from build123d import *

# Parameters (mm, degrees)
F1_DEPTH = 254
F2_DEPTH = 190.5
F3_DEPTH = 127
F4_DEPTH = 63.5
F5_R     = 12.6999
F6_R     = 25.3999
F7_R     = 12.6999


# Not quite as in the source:
# - a fillet or chamfer that OpenCascade refuses, or shapes differently, is made with other operations: its cross-section is extruded or revolved along the edge and cut away or added
# - a fillet or chamfer is up to 0.001 mm smaller than in the source, because OpenCascade refuses the exact size


with BuildPart() as f1:
    # F0 (on Right) → F1 (new body)
    with BuildSketch(Plane.YZ):
        with BuildLine():
            ThreePointArc((12.7, 0), (8.9802561211, 8.9802561211), (0, 12.7))
            ThreePointArc((0, 12.7), (-8.9802561211, 8.9802561211), (-12.7, 0))
            ThreePointArc((-12.7, 0), (-8.9802561211, -8.9802561211), (0, -12.7))
            ThreePointArc((0, -12.7), (8.9802561211, -8.9802561211), (12.7, 0))
        make_face()
    extrude(amount=F1_DEPTH)

    # F0 (on Right) → F2 (join)
    with BuildSketch(Plane.YZ):
        with BuildLine():
            ThreePointArc((-12.7, 0), (-8.9802561211, 8.9802561211), (0, 12.7))
            Line((0, 12.7), (-12.7, 12.7))
            Line((-12.7, 12.7), (-12.7, 0))
        make_face()
        with BuildLine():
            Line((12.7, 12.7), (0, 12.7))
            ThreePointArc((0, 12.7), (8.9802561211, 8.9802561211), (12.7, 0))
            Line((12.7, 0), (12.7, 12.7))
        make_face()
        with BuildLine():
            Line((12.7, -12.7), (12.7, 0))
            ThreePointArc((12.7, 0), (8.9802561211, -8.9802561211), (0, -12.7))
            Line((0, -12.7), (12.7, -12.7))
        make_face()
        with BuildLine():
            ThreePointArc((0, -12.7), (-8.9802561211, -8.9802561211), (-12.7, 0))
            Line((-12.7, 0), (-12.7, -12.7))
            Line((-12.7, -12.7), (0, -12.7))
        make_face()
    extrude(amount=F2_DEPTH)

    # F0 (on Right) → F3 (join)
    with BuildSketch(Plane.YZ):
        with BuildLine():
            ThreePointArc((25.4, 0), (17.9605122421, 17.9605122421), (0, 25.4))
            ThreePointArc((0, 25.4), (-17.9605122421, 17.9605122421), (-25.4, 0))
            ThreePointArc((-25.4, 0), (-17.9605122421, -17.9605122421), (0, -25.4))
            ThreePointArc((0, -25.4), (17.9605122421, -17.9605122421), (25.4, 0))
        make_face()
        Polygon((-12.7, 12.7), (0, 12.7), (12.7, 12.7), (12.7, 0), (12.7, -12.7), (0, -12.7), (-12.7, -12.7), (-12.7, 0), align=None, mode=Mode.SUBTRACT)
    extrude(amount=F3_DEPTH)

    # F0 (on Right) → F4 (join)
    with BuildSketch(Plane.YZ):
        with BuildLine():
            ThreePointArc((-25.4, 0), (-17.9605122421, 17.9605122421), (0, 25.4))
            Line((0, 25.4), (-25.4, 25.4))
            Line((-25.4, 25.4), (-25.4, 0))
        make_face()
        with BuildLine():
            ThreePointArc((0, -25.4), (-17.9605122421, -17.9605122421), (-25.4, 0))
            Line((-25.4, 0), (-25.4, -25.4))
            Line((-25.4, -25.4), (0, -25.4))
        make_face()
        with BuildLine():
            Line((25.4, -25.4), (25.4, 0))
            ThreePointArc((25.4, 0), (17.9605122421, -17.9605122421), (0, -25.4))
            Line((0, -25.4), (25.4, -25.4))
        make_face()
        with BuildLine():
            Line((25.4, 25.4), (0, 25.4))
            ThreePointArc((0, 25.4), (17.9605122421, 17.9605122421), (25.4, 0))
            Line((25.4, 0), (25.4, 25.4))
        make_face()
    extrude(amount=F4_DEPTH)

    # F5 (radius 12.7 in the source; OpenCascade refuses exactly that, so slightly less here)
    f5_edges = [f1.edges().sort_by_distance(p)[0] for p in [
        (158.75, -12.7, -12.7),
        (158.75, 12.7, -12.7),
        (158.75, 12.7, 12.7),
        (158.75, -12.7, 12.7),
    ]]
    fillet(f5_edges, radius=F5_R)

    # F6 (radius 25.4 in the source; OpenCascade refuses exactly that, so slightly less here)
    f6_edges = [f1.edges().sort_by_distance(p)[0] for p in [
        (31.75, -25.4, -25.4),
        (31.75, 25.4, -25.4),
        (31.75, -25.4, 25.4),
        (31.75, 25.4, 25.4),
    ]]
    fillet(f6_edges, radius=F6_R)

    # F7 (radius 12.7 in the source; OpenCascade refuses exactly that, so slightly less here)
    f7_edges = [f1.edges().sort_by_distance(p)[0] for p in [
        (127, 25.4, 0),
    ]]
    fillet(f7_edges, radius=F7_R)

    # F8: fillet of radius 6.35 on 1 edges, made by hand

    # F8_s1 → F8_t2 (revolve, cut)
    with BuildSketch(Plane.XY):
        with BuildLine():
            ThreePointArc((247.65, -12.7), (252.1401280605, -10.8401280605), (254, -6.35))
            Line((254, -6.35), (254, -12.7))
            Line((254, -12.7), (247.65, -12.7))
        make_face()
    revolve(axis=Axis((254, 0, 0), (-1, 0, 0)), mode=Mode.SUBTRACT)


solid = f1.part
Source: CAD feature listing. Evaluate the final solid. Frame: model axes, mm. A direction names the side the tool comes from. Give positions to 0.01 mm unless a question says otherwise; leave off trailing zeros. Write each loop counter-clockwise with the first axis right and the second up, starting at its lowest first coordinate (ties: lowest second). Pieces come first, ordered by that corner, then holes. Notation, with made-up numbers: (-11.75, 19.5) -> (-3.75, 19.5) arc R7 ccw to (-3.75, 24.5) -> close; hole circle Ø3 at (-6.5, 48.25). An arc over 180 degrees is marked (long way). Return JSON: item names as keys, results as strings. Group by question number.
1. Material intervals for line 1 (Z direction, x = 226, y = -11); line 2 (Y direction, x = 18, z = -0.5); line 3 (Y direction, x = 78.5, z = -22.5), sorted ascending. Write a range as from..to.
2. Section C-C, the plane x = 85. Output: boundary loops of the cut face in (y, z), then the cut area to 3 significant figures.
3. Section D-D, the plane x = 228.5. Output: boundary loops of the cut face in (y, z), then the cut area to 3 significant figures.
4. Access query for faces 1 (the face through (159.19, -8.88, -9.08)), 2 (the face through (159.19, -8.88, 9.08)), 3 (the face through (159.19, 9.08, 8.88)), 4 (the face through (159.19, 8.88, -9.08)). Directions: +Z, -Z, +X, -X, +Y, -Y. A direction counts if a zero-diameter tool reaches every point of the face in a straight line with its end or side. Return the directions, or none.
5. Pin query (flat end, axial travel): pin 1 Ø12 at (y, z) = (-12.5, 3.5) entering from +X; pin 2 Ø10 at (y, z) = (-15, 11) entering from +X; pin 3 Ø1 at (y, z) = (-19, -19.5) entering from +X; pin 4 Ø6 at (x, z) = (64, -19.5) entering from +Y. Return the tip coordinate at first contact, or that it passes through.
Determined:
{
 "1": {"line 1": "z = -6.35..6.35", "line 2": "y = -25.4..25.4", "line 3": "y = -11.79..11.79"},
 "2": {"outline": "circle Ø50.8 at (0, 0)", "area": "2,030 mm2"},
 "3": {"outline": "circle Ø25.4 at (0, 0)", "area": "507 mm2"},
 "4": {"face 1": "-Z, +X, -Y", "face 2": "+Z, +X, -Y", "face 3": "+Z, +X, +Y", "face 4": "-Z, +X, +Y"},
 "5": {"pin 1": "stops at x = 253.97", "pin 2": "stops at x = 126.97", "pin 3": "passes through", "pin 4": "stops at y = 19.31"}
}
